For this review, take the finished solid that the model builds, in its own axes (mm). A direction names the side the tool comes from. Coordinates: 2 decimals unless noted, no trailing zeros. Loops run counter-clockwise (first coordinate to the right, second up) from the corner with the lowest first, then second, coordinate; pieces in that order, holes last. Notation, with made-up numbers: M 9.5,-14.75 L 38.5,-14.75 A29 cw 38.5,24.25 Z; hole C 17.5,-8.75 d1. An arc over 180 degrees is marked long. Use one line per item in the form item = value.
```python
from build123d import *

# Parameters (mm, degrees)
SKETCH1_R           = 17.89
SKETCH1_R_2         = 4.075
SKETCH1_R_3         = 2.075
BOSS_EXTRUDE1_DEPTH = 3
BOSS_EXTRUDE2_START = 3
SKETCH1_4_R         = 4.075
SKETCH1_4_R_2       = 2.075
BOSS_EXTRUDE2_DEPTH = 5
BOSS_EXTRUDE3_START = 8
SKETCH1_5_R         = 4.075
SKETCH1_5_R_2       = 2.075
BOSS_EXTRUDE3_DEPTH = 5
FILLET1_R           = 2


with BuildPart() as part:
    # Sketch1 → Boss-Extrude1 (new body)
    # profile 1 of 3: a face of its own
    with BuildSketch(Plane(origin=(0, 0, 0), x_dir=(1, 0, 0), z_dir=(0, 1, 0))):
        with Locations(Location((-18.178896686, 33.907594253, 0), (0, 0, 270))):
            Circle(SKETCH1_R)
        with Locations((-18.178896686, 33.907594253)):
            Circle(SKETCH1_R_2, mode=Mode.SUBTRACT)
    # profile 2 of 3: a face of its own
    with BuildSketch(Plane(origin=(0, 0, 0), x_dir=(1, 0, 0), z_dir=(0, 1, 0))):
        with Locations((-18.178896686, 33.907594253)):
            Circle(SKETCH1_R_2)
        with Locations((-18.178896686, 33.907594253)):
            Circle(SKETCH1_R_3, mode=Mode.SUBTRACT)
    # profile 3 of 3: a face of its own
    with BuildSketch(Plane(origin=(0, 0, 0), x_dir=(1, 0, 0), z_dir=(0, 1, 0))):
        with Locations((-18.178896686, 33.907594253)):
            Circle(SKETCH1_R_3)
    extrude(amount=BOSS_EXTRUDE1_DEPTH)

    # Sketch1<4> → Boss-Extrude2 (add)
    # profile 1 of 2: a face of its own
    with BuildSketch(Plane(origin=(0, 0, 0), x_dir=(1, 0, 0), z_dir=(0, 1, 0)).offset(BOSS_EXTRUDE2_START)):
        with Locations(Location((-18.178896686, 33.907594253, 0), (0, 0, 270))):
            Circle(SKETCH1_4_R)
        with Locations((-18.178896686, 33.907594253)):
            Circle(SKETCH1_4_R_2, mode=Mode.SUBTRACT)
    # profile 2 of 2: a face of its own
    with BuildSketch(Plane(origin=(0, 0, 0), x_dir=(1, 0, 0), z_dir=(0, 1, 0)).offset(BOSS_EXTRUDE2_START)):
        with Locations((-18.178896686, 33.907594253)):
            Circle(SKETCH1_4_R_2)
    extrude(amount=BOSS_EXTRUDE2_DEPTH)

    # Sketch1<5> → Boss-Extrude3 (add)
    with BuildSketch(Plane(origin=(0, 0, 0), x_dir=(1, 0, 0), z_dir=(0, 1, 0)).offset(BOSS_EXTRUDE3_START)):
        with Locations(Location((-18.178896686, 33.907594253, 0), (0, 0, 270))):
            Circle(SKETCH1_5_R)
        with Locations(Location((-18.178896686, 33.907594253, 0), (0, 0, 270))):
            Circle(SKETCH1_5_R_2, mode=Mode.SUBTRACT)
    extrude(amount=BOSS_EXTRUDE3_DEPTH)

    # Fillet1
    fillet1_edges = [part.edges().sort_by_distance(p)[0] for p in [
        (-18.178896686, 13, -37.982594253),
        (-18.178896686, 3, -51.797594253),
    ]]
    fillet(fillet1_edges, radius=FILLET1_R - 0.0001)  # a hair under: the kernel refuses the full size


solid = part.part
```
1. Draft analysis for pull direction Z (two halves, no side actions). For faces 3 (the face through (-20.02, 10.46, -32.95)), 4 (the face through (-19.74, 6.944, -30.143)), 5 (the face through (-18, 8, -34)), 6 (the face through (-18, 0, -34)), state which applies: +Z half, -Z half, draft (parallel to the pull), parting line (faces both ways), or undercut.
Computed values:
face_3 = undercut
face_4 = parting line
face_5 = undercut
face_6 = draft
2. Consider section C-C on y = 8.5. Write out the cut boundary in (x, z) (3 decimals), plus the area to 3 significant figures.
Computed values:
outline = C -18.179,-33.908 d8.15; hole C -18.179,-33.908 d4.15
area = 38.6 mm2
3. Consider section B-B on y = 3.5. Write out the cut boundary in (x, z) (3 decimals), plus the area to 3 significant figures.
Computed values:
outline = C -18.179,-33.908 d8.15
area = 52.2 mm2
4. Tool access review of faces 1 (the face through (-21.5, 3, -30.6)), 2 (the face through (-34.05, 0.49, -25.65)): name each direction out of +Z, -Z, +X, -X, +Y, -Y from which nothing blocks a thin tool from reaching the whole face with its end or side.
Computed values:
face_1 = +Y
face_2 = +Y, -Y
5. Consider section D-D on y = 1.5. Write out the cut boundary in (x, z), plus the area to 3 significant figures.
Computed values:
outline = C -18.18,-33.91 d35.65
area = 998 mm2
6. For pin 1 Ø4 at (x, z) = (-5, -20.5) entering from +Y; pin 2 Ø2.5 at (x, z) = (-18.18, -33.91) entering from +Y; pin 3 Ø1 at (y, z) = (8, -28.5) entering from +X; pin 4 Ø5 at (x, z) = (-9.5, -42) entering from +Y, all flat-tipped, find the tip position at first contact; note any pin that passes through.
Computed values:
pin_1 = 2.78
pin_2 = 8
pin_3 = through
pin_4 = 3
7. Wall thickness on line 1 along Y through (x, z) = (-11, -31.5); line 2 along Z through (x, y) = (-17.5, 10); line 3 along X through (y, z) = (1.25, -19): over which ranges is each line inside the solid? List them lowest first. Write a range as from..to.
Computed values:
line_1 = 0..3
line_2 = -37.93..-35.87, -31.95..-29.89
line_3 = -28.04..-8.32
8. Consider section A-A on y = 11.5. Write out the cut boundary in (x, z) (3 decimals), plus the area to 3 significant figures.
Computed values:
outline = C -18.179,-33.908 d8.023; hole C -18.179,-33.908 d4.15
area = 37.0 mm2
